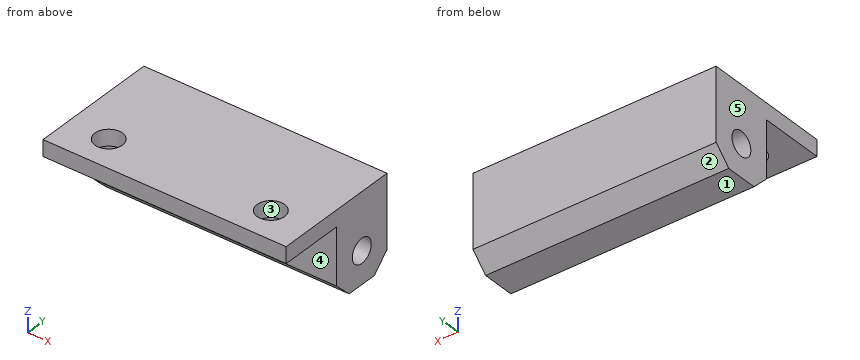
```python
from build123d import *

# Parameters (mm, degrees)
BOSS_EXTRUDE1_DEPTH     = 15
M3_CLEARANCE_HOLE1_D    = 3.4
SKETCH4_R               = 1.5
CUT_EXTRUDE1_DEPTH      = 1
CUT_EXTRUDE1_DEPTH_BACK = 31


with BuildPart() as part:
    # Sketch1 → Boss-Extrude1 (new body, symmetric)
    with BuildSketch(Plane(origin=(0, 0, 0), x_dir=(0, 0, -1), z_dir=(1, 0, 0))):
        Polygon((-7, 4), (2, 4), (4, 2), (4, -2), (2, -4), (-5, -4), (-5, -12), (-7, -12), align=None)
    extrude(amount=BOSS_EXTRUDE1_DEPTH, both=True)

    # M3 Clearance Hole1 (through all)
    with Locations(Plane(origin=(0, 0, 5), x_dir=(-1, 0, 0), z_dir=(0, 0, -1))):
        with Locations((-10, -8), (10, -8)):
            Hole(M3_CLEARANCE_HOLE1_D / 2)

    # Sketch4 → Cut-Extrude1 (cut, two sides)
    with BuildSketch(Plane(origin=(15, 0, 0), x_dir=(0, 0, -1), z_dir=(1, 0, 0))) as cut_extrude1_sk:
        Circle(SKETCH4_R)
    extrude(amount=CUT_EXTRUDE1_DEPTH, mode=Mode.SUBTRACT)
    extrude(cut_extrude1_sk.sketch, amount=-CUT_EXTRUDE1_DEPTH_BACK, mode=Mode.SUBTRACT)


solid = part.part
```
Model file for the job. Use its own axes, mm. Face numbers are marked on the shaded views. A direction names the side the tool comes from. Coordinates: 2 decimals unless noted, no trailing zeros. Loops run counter-clockwise (first coordinate to the right, second up) from the corner with the lowest first, then second, coordinate; pieces in that order, holes last. Notation, with made-up numbers: (53, -1) - (88, -1) arc R25 cw to (88, 19) - close; hole circle Ø8 at (14.25, -28). An arc over 180 degrees is marked (long way). Answer as a JSON object with one key per item and string values. Group by question number.
(1) Flat gauge pins, fed straight in: pin 1 (6 mm diameter, centred on x = -5, z = 0.5, fed in from -Y); pin 2 (4 mm diameter, centred on x = 6.5, y = -9, fed in from -Z). Where does each tip first touch, or does it go through?
(2) Tool access for the marked faces 4 and 5: list every direction of +Z, -Z, +X, -X, +Y, -Y with a clear straight run to the whole face (end or side of a thin tool).
(3) Cut at D-D (x = 2.25). Give the cut face in (y, z).
(4) Cut at C-C (z = 0). Give the cut face in (x, y).
(5) Cut at A-A (x = 10). Give the cut face in (y, z).
(6) Cut at B-B (y = -8). Give the cut face in (x, z).
(7) Probe line 1 along Y through (x, z) = (8.25, 0); line 2 along X through (y, z) = (-8.75, 6.5); line 3 along Y through (x, z) = (10, 5.85). List the from-to ranges inside material, lowest first.
(8) Two-plate mould, pull along Y, no slides. Class the marked faces 1, 2 and 3: released by +Y, released by -Y, zero draft, split by the parting line, or undercut.
Geometry says:
{
 "1": {"pin 1": "stops at y = -4", "pin 2": "stops at z = 5"},
 "2": {"face 4": "-Z, +X, -X, -Y", "face 5": "+Z, -Z, -X, +Y, -Y"},
 "3": {"outline": "(-12, 5) - (-4, 5) - (-4, -2) - (-2, -4) - (2, -4) - (4, -2) - (4, 7) - (-12, 7) - close; hole circle Ø3 at (0, 0)"},
 "4": {"outline": "(-15, -4) - (15, -4) - (15, -1.5) - (-15, -1.5) - close; (-15, 1.5) - (15, 1.5) - (15, 4) - (-15, 4) - close"},
 "5": {"outline": "(-12, 5) - (-9.7, 5) - (-9.7, 7) - (-12, 7) - close; (-6.3, 5) - (-4, 5) - (-4, -2) - (-2, -4) - (2, -4) - (4, -2) - (4, 7) - (-6.3, 7) - close; hole circle Ø3 at (0, 0)"},
 "6": {"outline": "(-15, 5) - (-11.7, 5) - (-11.7, 7) - (-15, 7) - close; (-8.3, 5) - (8.3, 5) - (8.3, 7) - (-8.3, 7) - close; (11.7, 5) - (15, 5) - (15, 7) - (11.7, 7) - close"},
 "7": {"line 1": "y = -4 to -1.5, 1.5 to 4", "line 2": "x = -15 to -11.53, -8.47 to 8.47, 11.53 to 15", "line 3": "y = -12 to -9.7, -6.3 to 4"},
 "8": {"face 1": "zero draft", "face 2": "released by +Y", "face 3": "undercut"}
}
